Autodesk Inventor part; units mm, degrees
ref_plane "YZ Plane" through (0, 0, 0) normal (1, 0, 0) x (0, 1, 0)
ref_plane "XZ Plane" through (0, 0, 0) normal (0, 1, 0) x (-1, 0, 0)
ref_plane "XY Plane" through (0, 0, 0) normal (0, 0, 1) x (1, 0, 0)
sketch "Sketch1" plane through (0, 0, 0) normal (0, 1, 0) x (-1, 0, 0)
  line L0 (0, 0) -> (-25.4, 0)
  line L1 (-25.4, -152.4) -> (-157.48, -152.4)
  line L2 (-157.48, -152.4) -> (-157.48, -177.8)
  line L3 (-157.48, -177.8) -> (0, -177.8)
  line L4 (0, -177.8) -> (0, -152.4)
  line L5 (-25.4, -152.4) -> (0, -152.4)
  dimension "d2" = 25.4
  dimension "d23" = 157.48
extrude "Extrusion1" add sketch "Sketch1" along normal blind 25.4
sketch "Sketch2" plane through (0, 25.4, 0) normal (0, 1, 0) x (1, 0, 0)
  circle A0 centre (144.78, 165.1) radius 6.35
  line L0 (157.48, 152.4) -> (157.48, 177.8)
  line L1 (157.48, 177.8) -> (0, 177.8)
  circle A1 centre (12.7, 165.1) radius 6.35
  line L2 (0, 152.4) -> (157.48, 152.4)
  line L3 (0, 177.8) -> (0, 152.4)
  point P0 (0, 0)
  dimension "d5" = 12.7
  dimension "d6" = 12.7
  dimension "d7" = 12.7
  dimension "d16" = 12.7
  dimension "d17" = 12.7
extrude "Extrusion2" cut sketch "Sketch2" against normal blind 41.275 contours A0 | A1
fillet "Fillet1" radius 12.7 4 edges at (157.48, 12.7, -152.4) (157.48, 12.7, -177.8) (0, 12.7, -152.4) (0, 12.7, -177.8)
sketch "Sketch4" plane through (0, 0, 0) normal (0, -1, 0) x (1, 0, 0)
  circle A0 centre (106.68, -165.1) radius 3.175
  line L0 (144.78, -177.8) -> (12.7, -177.8)
  circle A1 centre (144.78, -165.1) radius 6.35
  point P0 (0, 0)
  dimension "d18" = 6.35
  dimension "d19" = 12.7
  dimension "d20" = 38.1
extrude "Extrusion4" add sketch "Sketch4" along normal blind 25.4 contours A0
properties part number "arm" material "Aluminum 6061"
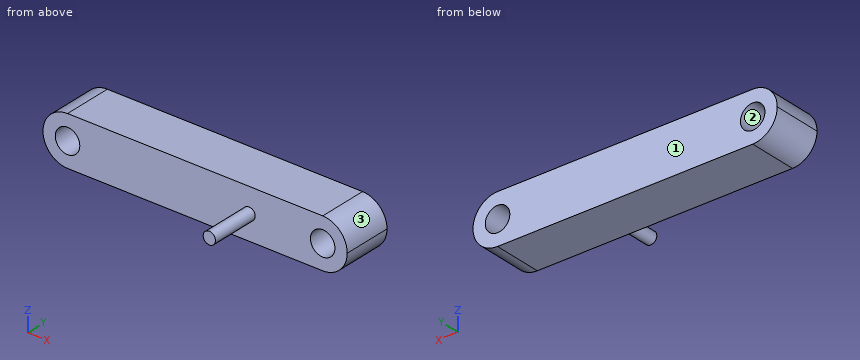
Here's how the part is built. I have some questions about the finished solid (model axes, mm). Face numbers are marked on the shaded views. Coordinates: 2 decimals unless noted, no trailing zeros. Order: outer loops, then holes, each group sorted by start corner. A loop starts at its lowest first (then second) coordinate and runs counter-clockwise, first axis right, second up. Notation, with made-up numbers: M -25,71 L 22,71 A31 ccw 22,109 Z; hole C 24,12 d4. An arc over 180 degrees is marked long. Answer as a JSON object with one key per item and string values. Group by question number.
(1) Suppose I cut it at C-C, the plane x = 142.5. Please give me the cut outline in (y, z).
(2) For pin 1 (1 mm diameter, centred on y = -8.5, z = -164, fed in from -X); pin 2 (3 mm diameter, centred on y = -1, z = -172, fed in from +X); pin 3 (8 mm diameter, centred on x = 115.5, z = -174.5, fed in from -Y), each with a flat end and sliding along its axis, tell me the tip position at first contact or that it passes through.
(3) Suppose I cut it at D-D, the plane y = -15. Please give me the cut outline in (x, z) (3 decimals), then the cut area to 3 significant figures.
(4) If we mould it in two halves opening along X, with no side actions, what happens to the marked faces 1, 2 and 3? For each: released by +X, released by -X, zero draft, split by the parting line, or undercut.
(5) Suppose I cut it at B-B, the plane x = 106.68. Please give me the cut outline in (y, z) (3 decimals), then the cut area to 3 significant figures.
(6) Suppose I cut it at A-A, the plane y = 20. State how many separate pieces and enclosed holes the cut face has, then the cut area to 3 significant figures.
(7) I need wall thicknesses on probe 1 along X at (y, z) = (10.5, -165.1); probe 2 along Z at (x, y) = (144.78, 7.5); probe 3 along X at (y, z) = (7, -169). Which ranges of each line are inside material? Lowest first, please.
Values found:
{
 "1": {"outline": "M 0,-177.8 L 25.4,-177.8 L 25.4,-171.03 L 0,-171.03 Z; M 0,-159.17 L 25.4,-159.17 L 25.4,-152.4 L 0,-152.4 Z"},
 "2": {"pin 1": "stops at x = 103.56", "pin 2": "stops at x = 156.09", "pin 3": "stops at y = 0"},
 "3": {"outline": "C 106.68,-165.1 d6.35", "area": "31.7 mm^2"},
 "4": {"face 1": "zero draft", "face 2": "undercut", "face 3": "released by +X"},
 "5": {"outline": "M -25.4,-168.275 L 0,-168.275 L 0,-177.8 L 25.4,-177.8 L 25.4,-152.4 L 0,-152.4 L 0,-161.925 L -25.4,-161.925 Z", "area": "806 mm^2"},
 "6": {"separate pieces": "1", "enclosed holes": "2", "area": "3,610 mm^2"},
 "7": {"probe 1": "x = 0 to 6.35, 19.05 to 138.43, 151.13 to 157.48", "probe 2": "z = -177.8 to -171.45, -158.75 to -152.4", "probe 3": "x = 0.61 to 7.69, 17.71 to 139.77, 149.79 to 156.87"}
}
